Input: dimensioned drawing with shaded views. Units: mm. Origin: part minimum x, y, z. Round coordinates to 2 decimals unless told otherwise and drop trailing zeros. Loops run counter-clockwise (first coordinate to the right, second up) from the corner with the lowest first, then second, coordinate; pieces in that order, holes last. Notation, with made-up numbers: M 0,29 L 19,29 A22 ccw 19,53 Z; hole C 50,88 d1. An arc over 180 degrees is marked long. Use one line per item in the form item = value. Start each with the question number.
Q1. Section query C-C, the plane z = 0.45. Output: boundary loops of the cut face in (x, y), and give its area (3 significant figures).
Q2. Section query D-D, the plane x = 2. Output: boundary loops of the cut face in (y, z), and give its area (3 significant figures).
Q3. Section query A-A, the plane y = 10. Output: boundary loops of the cut face in (x, z).
Q4. First-contact query: P1, Ø2.5, axis at x = 5.5, z = 4, coming from the +Y side; P2, Ø1, axis at y = 4.5, z = 4, coming from the +X side; P3, Ø1.5, axis at y = 2.5, z = 4, coming from the +X side; P4, Ø2.5, axis at x = 10, y = 10, coming from the -Z side. Flat tips, straight axial feed; report the tip coordinate or a pass-through.
Q5. Ray query, line 1 along Y through (x, z) = (10, 1.3); line 2 along Y through (x, z) = (6.5, 2.4); line 3 along X through (y, z) = (10.5, 2) (1 decimal). Return the intervals inside material, ascending.
Q6. Mould query, pull axis X, two halves, no side actions, for the marked faces 1, 2 and 3. Classes: pulls with the +X half, pulls with the -X half, needs draft (parallel to the pull), parting line crosses it, or undercut.
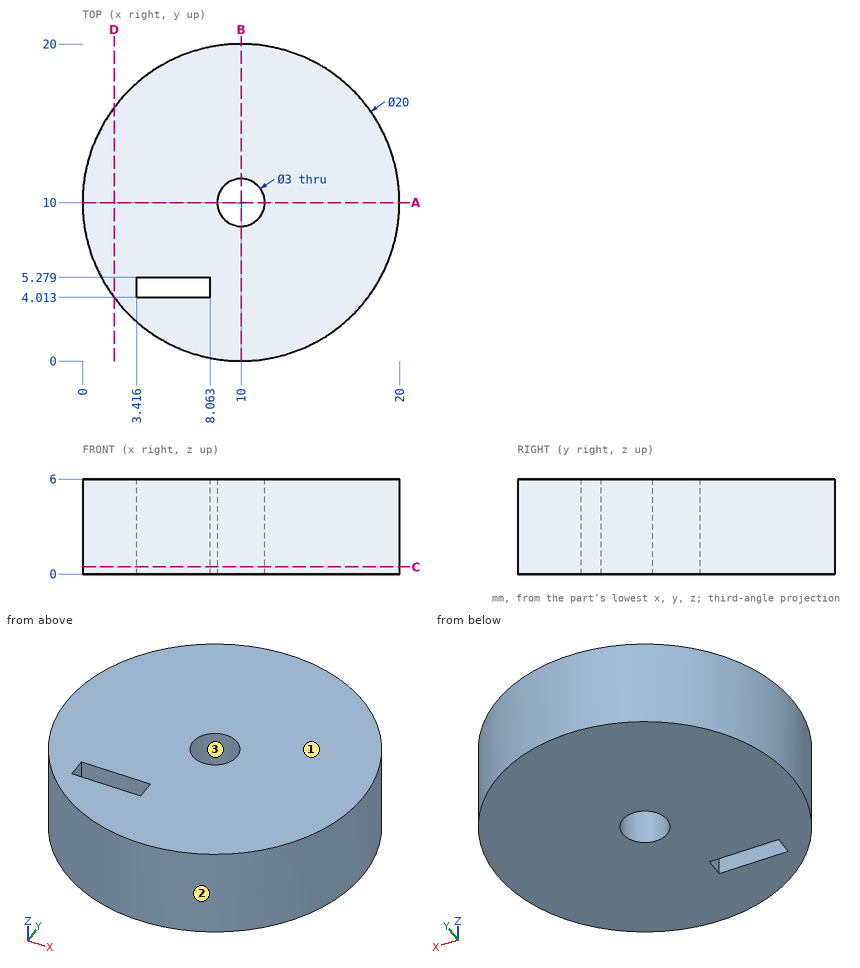
Results found:
q1.outline = C 10,10 d20; hole M 3.42,4.01 L 8.06,4.01 L 8.06,5.28 L 3.42,5.28 Z; hole C 10,10 d3
q1.area = 301 mm²
q2.outline = M 4,0 L 16,0 L 16,6 L 4,6 Z
q2.area = 72.0 mm²
q3.outline = M 0,0 L 8.5,0 L 8.5,6 L 0,6 Z; M 11.5,0 L 20,0 L 20,6 L 11.5,6 Z
q4.P1 = 19.46
q4.P2 = 18.66
q4.P3 = 17.38
q4.P4 = through
q5.line_1 = 0 to 8.5, 11.5 to 20
q5.line_2 = 0.63 to 4.01, 5.28 to 19.37
q5.line_3 = 0 to 8.6, 11.4 to 20
q6.face_1 = needs draft
q6.face_2 = parting line crosses it
q6.face_3 = undercut
